from build123d import *

# Parameters (mm, degrees)
SKETCH1_W                 = 35.814
SKETCH1_H                 = 7.62
BOSS_EXTRUDE1_DEPTH       = 8.636
SKETCH4_W                 = 8.89
SKETCH4_H                 = 1.778
CUT_EXTRUDE1_DEPTH        = 8.62
SKETCH6_W                 = 8.255
SKETCH6_H                 = 7.366
CUT_EXTRUDE2_DEPTH        = 8.62
SKETCH7_R                 = 2.159
CUT_EXTRUDE3_DEPTH        = 7.858
CUT_EXTRUDE4_REACH        = 10.636
SKETCH8_R                 = 2.159
F_6_32_TAPPED_HOLE1_D     = 2.7051
F_6_32_TAPPED_HOLE1_DEPTH = 0.635


with BuildPart() as part:
    # Sketch1 → Boss-Extrude1 (new body)
    with BuildSketch(Plane.XY):
        with Locations((-21.190085106, 0.628244681)):
            Rectangle(SKETCH1_W, SKETCH1_H)
    extrude(amount=BOSS_EXTRUDE1_DEPTH)

    # Sketch4 → Cut-Extrude1 (cut, through all)
    with BuildSketch(Plane(origin=(0, 4.438244681, 0), x_dir=(1, 0, 0), z_dir=(0, 1, 0))):
        with Locations((-34.652085106, -0.889)):
            Rectangle(SKETCH4_W, SKETCH4_H)
        with Locations((-34.652085106, -7.747)):
            Rectangle(SKETCH4_W, SKETCH4_H)
    extrude(amount=-CUT_EXTRUDE1_DEPTH, mode=Mode.SUBTRACT)

    # Sketch6 → Cut-Extrude2 (cut, through all)
    with BuildSketch(Plane(origin=(0, 4.438244681, 0), x_dir=(1, 0, 0), z_dir=(0, 1, 0))):
        with Locations((-7.410585106, -4.318)):
            Rectangle(SKETCH6_W, SKETCH6_H)
    extrude(amount=-CUT_EXTRUDE2_DEPTH, mode=Mode.SUBTRACT)

    # Sketch7 → Cut-Extrude3 (cut, through all)
    with BuildSketch(Plane.XY.offset(6.858)):
        with Locations((-35.287085106, 0.628244681)):
            Circle(SKETCH7_R)
    extrude(amount=-CUT_EXTRUDE3_DEPTH, mode=Mode.SUBTRACT)

    # Sketch8 → Cut-Extrude4 (cut, up to next)
    with BuildSketch(Plane.XY.offset(8.636), mode=Mode.PRIVATE) as cut_extrude4_sk1:
        with Locations((-7.093085106, 0.628244681)):
            Circle(SKETCH8_R)
    cut_extrude4_tool1 = extrude(cut_extrude4_sk1.sketch, amount=-CUT_EXTRUDE4_REACH, mode=Mode.PRIVATE) & part.part
    add(cut_extrude4_tool1.solids().sort_by_distance((-7.093085, 0.628245, 8.636))[0], mode=Mode.SUBTRACT)

    # #6-32 Tapped Hole1
    with Locations(Plane(origin=(0, 0, 0), x_dir=(-1, 0, 0), z_dir=(0, 0, -1))):
        with Locations((7.093085106, 0.628244681)):
            Hole(F_6_32_TAPPED_HOLE1_D / 2, depth=F_6_32_TAPPED_HOLE1_DEPTH)


solid = part.part
Work out the finished part from the listing and answer in its coordinate system (mm). A direction names the side the tool comes from. Give positions to 0.01 mm unless a question says otherwise; leave off trailing zeros. Order: outer loops, then holes, each group sorted by start corner. A loop starts at its lowest first (then second) coordinate and runs counter-clockwise, first axis right, second up. Notation, with made-up numbers: M 53,-16.5 L 84,-16.5 A14 cw 84,-5.5 Z; hole C -16,7 d4. An arc over 180 degrees is marked long. Return JSON: item names as keys, results as strings.
Q1. Find section C-C, the plane z = 3. Write down the section's boundary in (x, y), and give its area (3 significant figures).
Answer below:
{"outline": "M -39.1,-3.18 L -11.54,-3.18 L -11.54,4.44 L -39.1,4.44 Z; hole C -35.29,0.63 d4.32", "area": "195 mm^2"}
Q2. Find section D-D, the plane x = -35.5. Write down the section's boundary in (y, z).
Answer below:
{"outline": "M -3.18,1.78 L -1.52,1.78 L -1.52,6.86 L -3.18,6.86 Z; M 2.78,1.78 L 4.44,1.78 L 4.44,6.86 L 2.78,6.86 Z"}
Q3. Which of the six approach directions +Z, -Z, +X, -X, +Y, -Y give full straight-line access (tool end or side, diameter ignored) to faces 1 (the face through (-8.4, -0.2, 0.635)), 2 (the face through (-30.207, 1, 1)), 3 (the face through (-39.097, 1, 4)), 4 (the face through (-33, 1, 6.858))?
Answer below:
{"face 1": "+X, +Y, -Y", "face 2": "-Z, -X, +Y, -Y", "face 3": "+Z, -Z, -X, +Y, -Y", "face 4": "+Z, -X, +Y, -Y"}
Q4. Find section B-B, the plane y = 1.25. Write down the section's boundary in (x, z) (3 decimals), and give its area (3 significant figures).
Answer below:
{"outline": "M -39.097,1.778 L -37.355,1.778 L -37.355,6.858 L -39.097,6.858 Z; M -33.22,1.778 L -30.207,1.778 L -30.207,0 L -8.294,0 L -8.294,0.635 L -11.538,0.635 L -11.538,8.001 L -9.161,8.001 L -9.161,8.636 L -30.207,8.636 L -30.207,6.858 L -33.22,6.858 Z; M -5.892,0 L -3.283,0 L -3.283,0.635 L -5.892,0.635 Z; M -5.026,8.001 L -3.283,8.001 L -3.283,8.636 L -5.026,8.636 Z", "area": "192 mm^2"}
Q5. Find the intervals of material crossed by line 1 along Z through (x, y) = (-5.5, -1.5) (3 decimals); line 2 along Z through (x, y) = (-33, 0.75); line 3 along X through (y, z) = (0.75, 4.25), in increasing order. Write a range as [from, to].
Answer below:
{"line 1": "z = [0, 0.635], [8.001, 8.636]", "line 2": "z = [1.78, 6.86]", "line 3": "x = [-39.1, -37.44], [-33.13, -11.54]"}
Q6. The mould has two halves that part along X. Classify faces 5 (the face through (-30.207, 1, 8)), 6 (the face through (-36.878, 2.087, 4.354)), 7 (the face through (-17, 1, 0)), 8 (the face through (-5.034, 1.277, 8.323)): pulls with the +X half, pulls with the -X half, needs draft (parallel to the pull), parting line crosses it, or undercut.
Answer below:
{"face 5": "pulls with the -X half", "face 6": "undercut", "face 7": "needs draft", "face 8": "undercut"}
Q7. Find section A-A, the plane x = -11. Write down the section's boundary in (y, z) (3 decimals).
Answer below:
{"outline": "M -3.182,0 L 4.438,0 L 4.438,0.635 L -3.182,0.635 Z; M -3.182,8.001 L 4.438,8.001 L 4.438,8.636 L -3.182,8.636 Z"}
Q8. Each of these flat-tipped pins is pushed along its axis until it touches: pin 1 (4 mm diameter, centred on x = -14, y = 2.5, fed in from -Z); pin 2 (2.5 mm diameter, centred on x = -36.5, y = 1.5, fed in from -Z); pin 3 (0.9 mm diameter, centred on y = 1.5, z = 7.5, fed in from -X); pin 4 (3.5 mm diameter, centred on y = 0.5, z = 5.5, fed in from +X). Where does it stop, or does it pass through?
Answer below:
{"pin 1": "stops at z = 0", "pin 2": "stops at z = 1.78", "pin 3": "stops at x = -30.21", "pin 4": "stops at x = -11.54"}
